Input: dimensioned drawing with shaded views. Units: mm. Origin: part minimum x, y, z. Give positions to 0.01 mm unless a question says otherwise; leave off trailing zeros. Loops run counter-clockwise (first coordinate to the right, second up) from the corner with the lowest first, then second, coordinate; pieces in that order, holes last. Notation, with made-up numbers: M 67,41.5 L 99,41.5 A23 cw 99,67.5 Z; hole C -4,-26 d10. An arc over 180 degrees is marked long. Use CSV: the item, a comma, the result in double quotes. Start each with the question number.
Q1. Section D-D, the plane z = 72. Output: boundary loops of the cut face in (x, y).
Q2. Material intervals for line 1 along X through (y, z) = (3.6, 16); line 2 along Z through (x, y) = (48, 2.85); line 3 along Z through (x, y) = (4, 1.1), sorted ascending.
Q3. Section A-A, the plane x = 3. Output: boundary loops of the cut face in (y, z), plus the area to 3 significant figures.
Q4. Section C-C, the plane y = 0.75. Output: boundary loops of the cut face in (x, z).
Q5. Pin query (flat end, axial travel): pin 1 (4 mm diameter, centred on x = 48, z = 61, fed in from -Y); pin 2 (1.8 mm diameter, centred on x = 3, z = 61, fed in from +Y). Return the tip coordinate at first contact, or that it passes through.
Q6. Section B-B, the plane z = 61. Output: boundary loops of the cut face in (x, y), plus the area to 3 significant figures.
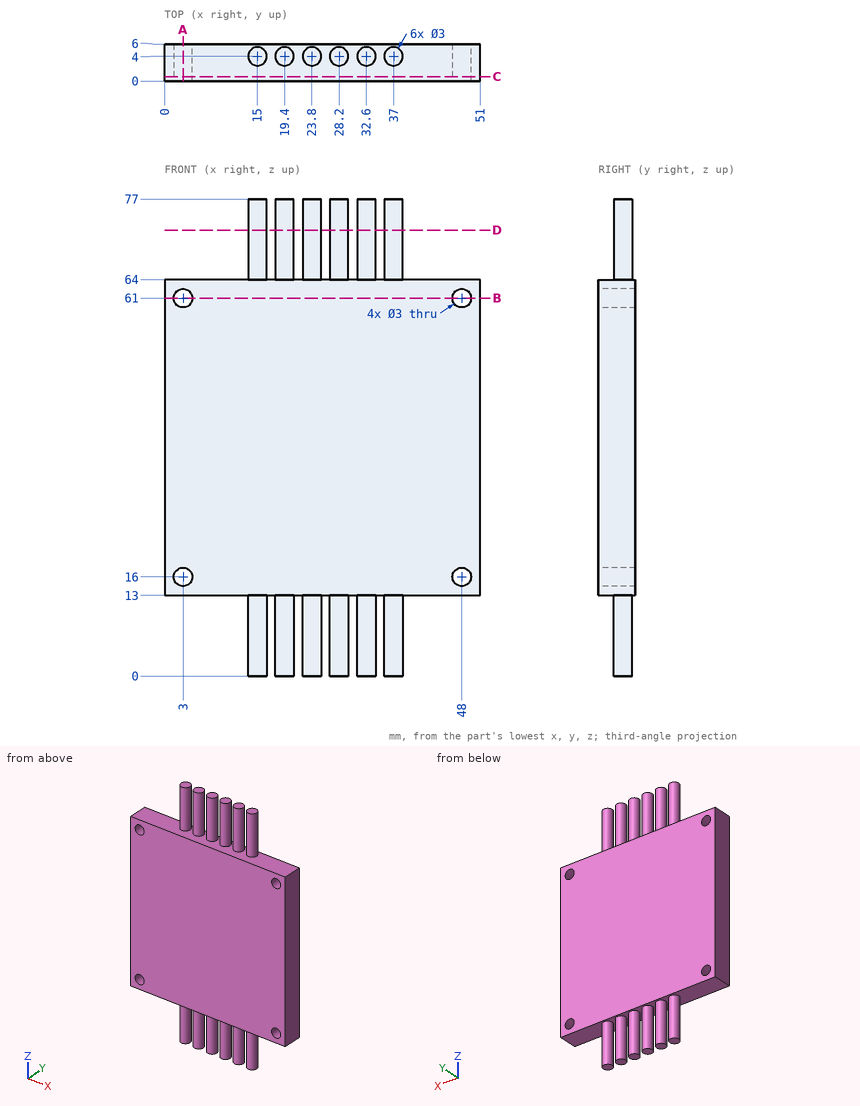
A:
1,outline,"C 15,4 d3; C 19.4,4 d3; C 23.8,4 d3; C 28.2,4 d3; C 32.6,4 d3; C 37,4 d3"
2,line 1,"0 to 1.5, 4.5 to 46.5, 49.5 to 51"
2,line 2,"13 to 14.5, 17.5 to 59.5, 62.5 to 64"
2,line 3,"13 to 14.88, 17.12 to 59.88, 62.12 to 64"
3,outline,"M 0,13 L 6,13 L 6,14.5 L 0,14.5 Z; M 0,17.5 L 6,17.5 L 6,59.5 L 0,59.5 Z; M 0,62.5 L 6,62.5 L 6,64 L 0,64 Z"
3,area,"270 mm^2"
4,outline,"M 0,13 L 51,13 L 51,64 L 0,64 Z; hole C 3,16 d3; hole C 3,61 d3; hole C 48,16 d3; hole C 48,61 d3"
5,pin 1,"y = 0"
5,pin 2,"through"
6,outline,"M 0,0 L 1.5,0 L 1.5,6 L 0,6 Z; M 4.5,0 L 46.5,0 L 46.5,6 L 4.5,6 Z; M 49.5,0 L 51,0 L 51,6 L 49.5,6 Z"
6,area,"270 mm^2"
